from build123d import *

# Parameters (mm, degrees)
CROQUIS1_R              = 17.5
CROQUIS1_R_2            = 12.5
SALIENTE_EXTRUIR1_DEPTH = 40
CROQUIS2_W              = 35
CROQUIS2_H              = 40
SALIENTE_EXTRUIR2_DEPTH = 30
CORTAR_EXTRUIR1_START   = -55
CROQUIS3_R              = 12.5
CORTAR_EXTRUIR1_DEPTH   = 55
CROQUIS4_W              = 26
CROQUIS4_H              = 10
CORTAR_EXTRUIR2_DEPTH   = 55
CROQUIS5_R              = 2.5
CORTAR_EXTRUIR3_DEPTH   = 55
CHAFL_N1_SIZE           = 5
CHAFL_N1_SIZE_2         = 11.23018387
CROQUIS6_W              = 43.374633734
CROQUIS6_H              = 44.438316851
CORTAR_EXTRUIR4_DEPTH   = 5.5
CROQUIS7_R              = 5.5
CORTAR_EXTRUIR5_DEPTH   = 4


with BuildPart() as part:
    # Croquis1 → Saliente-Extruir1 (new body)
    with BuildSketch(Plane(origin=(0, 0, 0), x_dir=(1, 0, 0), z_dir=(0, 1, 0))):
        with Locations(Location((0, 0, 0), (0, 0, 270))):
            Circle(CROQUIS1_R)
        with Locations(Location((0, 0, 0), (0, 0, 270))):
            Circle(CROQUIS1_R_2, mode=Mode.SUBTRACT)
    extrude(amount=SALIENTE_EXTRUIR1_DEPTH)

    # Croquis2 → Saliente-Extruir2 (add)
    with BuildSketch(Plane.XY):
        with Locations((0, 20)):
            Rectangle(CROQUIS2_W, CROQUIS2_H)
    extrude(amount=SALIENTE_EXTRUIR2_DEPTH)

    # Croquis3 → Cortar-Extruir1 (cut)
    with BuildSketch(Plane(origin=(0, 40, 0), x_dir=(1, 0, 0), z_dir=(0, 1, 0)).offset(CORTAR_EXTRUIR1_START)):
        with Locations(Location((0, 0, 0), (0, 0, 270))):
            Circle(CROQUIS3_R)
    extrude(amount=CORTAR_EXTRUIR1_DEPTH, mode=Mode.SUBTRACT)

    # Croquis4 → Cortar-Extruir2 (cut)
    with BuildSketch(Plane(origin=(0, 40, 0), x_dir=(1, 0, 0), z_dir=(0, 1, 0))):
        with Locations((0, -19.512798854)):
            Rectangle(CROQUIS4_W, CROQUIS4_H)
    extrude(amount=-CORTAR_EXTRUIR2_DEPTH, mode=Mode.SUBTRACT)

    # Croquis5 → Cortar-Extruir3 (cut)
    with BuildSketch(Plane.XY.offset(30)):
        with Locations((16, 18)):
            Circle(CROQUIS5_R)
        with Locations((-16, 18)):
            Circle(CROQUIS5_R)
    extrude(amount=-CORTAR_EXTRUIR3_DEPTH, mode=Mode.SUBTRACT)

    # Chaflán1
    # the kernel refuses this chamfer: 11.23018387, 5 mm, written as the material it takes off along each edge
    with BuildSketch(Plane(origin=(17.5, 40, 0), x_dir=(-0.9968798599783936, 0.07893379991777015, 0), z_dir=(0, 0, 1))) as chafl_n1_piece_1:
        Polygon((CHAFL_N1_SIZE * 0.996879859978, CHAFL_N1_SIZE * 0.0789337999178), (-CHAFL_N1_SIZE_2 * 0.0789337999144, CHAFL_N1_SIZE_2 * 0.996879859936), (0, 0), align=None)
    extrude(amount=59.104972531, mode=Mode.SUBTRACT)
    with BuildSketch(Plane(origin=(-17.5, 40, 0), x_dir=(0.9968798599783936, 0.07893379991777015, 0), z_dir=(0, 0, 1))) as chafl_n1_piece_2:
        Polygon((CHAFL_N1_SIZE * 0.996879859978, -CHAFL_N1_SIZE * 0.0789337999178), (-CHAFL_N1_SIZE_2 * 0.0789337999144, -CHAFL_N1_SIZE_2 * 0.996879859936), (0, 0), align=None)
    extrude(amount=59.104972531, mode=Mode.SUBTRACT)
    with BuildSketch(Plane(origin=(0, 40, 0), x_dir=(1, 0, 0), z_dir=(0, 0, 1))) as chafl_n1_piece_3:
        Polygon((17.5 - CHAFL_N1_SIZE, 0), (17.5, -CHAFL_N1_SIZE_2), (17.5, 0), align=None)
    revolve(axis=Axis((0, 40, 0), (0, 1, 0)), revolution_arc=180, mode=Mode.SUBTRACT)

    # Croquis6 → Cortar-Extruir4 (cut)
    with BuildSketch(Plane.XY.offset(30)):
        with Locations((0, 20.325014285)):
            Rectangle(CROQUIS6_W, CROQUIS6_H)
    extrude(amount=-CORTAR_EXTRUIR4_DEPTH, mode=Mode.SUBTRACT)

    # Croquis7 → Cortar-Extruir5 (cut)
    with BuildSketch(Plane.XY.offset(14)):
        with Locations((-16, 18)):
            Circle(CROQUIS7_R)
    cortar_extruir5 = extrude(amount=-CORTAR_EXTRUIR5_DEPTH, mode=Mode.SUBTRACT)

    # Simetría1: Cortar-Extruir5 across plane
    add(cortar_extruir5.mirror(Plane(origin=(0, 0, 0), x_dir=(0, 0, 1), z_dir=(1, 0, 0))), mode=Mode.SUBTRACT)


solid = part.part
For this review, take the finished solid that the model builds, in its own axes (mm). A direction names the side the tool comes from. Round coordinates to 2 decimals unless told otherwise and drop trailing zeros. Order: outer loops, then holes, each group sorted by start corner. A loop starts at its lowest first (then second) coordinate and runs counter-clockwise, first axis right, second up. Notation, with made-up numbers: M 56.25,19.25 L 90.25,19.25 A36 cw 90.25,53.25 Z; hole C 75,66.5 d2. An arc over 180 degrees is marked long. Use a Markdown table: item, result. Add a question column.
Item 1: To check wall thickness, follow line 1 along X through (y, z) = (9.5, 0); line 2 along X through (y, z) = (24.5, 17); line 3 along Y through (x, z) = (-16, 21). State the ranges of each line that lie inside material, in increasing order.
Item 2: Add section A-A, the plane z = 19. Give the boundary of the cut face in (x, y).
Item 3: Mouldability with a two-part tool opening along X and no side actions: class faces 4 (the conical face through (0.31, 36.8, -13.92)), 5 (the flat face through (-13, 20, 20)), 6 (the flat face through (17.5, 8, 12)) as released by +X, released by -X, zero draft, split by the parting line, or undercut.
Item 4: Add section C-C, the plane y = 18. Give the boundary of the cut face in (x, z).
Item 5: Add section D-D, the plane z = 1.5. Give the boundary of the cut face in (x, y), then the cut area to 3 significant figures.
Item 6: Tool access review of faces 1 (the cylindrical face through (-10.5, 17.9, 12)), 2 (the flat face through (-17.5, 8, 12)), 3 (the flat face through (13, 20, 20)): name each direction out of +Z, -Z, +X, -X, +Y, -Y from which nothing blocks a thin tool from reaching the whole face with its end or side.
Item 7: Insertion check: pin 1 (12 mm diameter, centred on x = -9.5, z = 18, fed in from +Y); pin 2 (5.5 mm diameter, centred on x = -13, y = 16.5, fed in from -Z); pin 3 (4.5 mm diameter, centred on x = -16, y = 18, fed in from +Z) (3 decimals); pin 4 (13 mm diameter, centred on x = 6, y = 27.5, fed in from +Z). Each pin has a flat end and moves straight along its axis. Give the tip position at first contact, or say it passes through.
Item 8: Add section B-B, the plane x = 0. Give the boundary of the cut face in (y, z).
Geometry results:
| question | item | result |
|---|---|---|
| 1 | line 1 | x = -17.5 to -12.5, 12.5 to 17.5 |
| 1 | line 2 | x = -17.5 to -13, 13 to 17.5 |
| 1 | line 3 | y = 0 to 15.5, 20.5 to 32.14 |
| 2 | outline | M -17.5,0 L -13,0 L -13,38.88 L -17.5,28.77 L -17.5,20 A2.5 cw long -17.5,16 Z; M 13,0 L 17.5,0 L 17.5,16 A2.5 cw long 17.5,20 L 17.5,28.77 L 13,38.88 Z |
| 3 | face 4 | split by the parting line |
| 3 | face 5 | undercut |
| 3 | face 6 | released by +X |
| 4 | outline | M -13.5,-11.14 A17.5 ccw 13.5,-11.14 L 13.5,10 L 10.5,10 L 10.5,14 L 13.5,14 L 13.5,24.5 L 13,24.5 L 13,14.51 L -13,14.51 L -13,24.5 L -13.5,24.5 L -13.5,14 L -10.5,14 L -10.5,10 L -13.5,10 Z; hole C 0,0 d25 |
| 5 | outline | M -17.5,0 L -12.41,0 L -12.41,40 L -12.5,40 L -17.5,28.77 L -17.5,20 A2.5 cw long -17.5,16 Z; M 12.41,0 L 17.5,0 L 17.5,16 A2.5 cw long 17.5,20 L 17.5,28.77 L 12.5,40 L 12.41,40 Z |
| 5 | area | 317 mm² |
| 6 | face 1 | none |
| 6 | face 2 | +Z, -Z, -X, +Y, -Y |
| 6 | face 3 | +Z, +Y, -Y |
| 7 | pin 1 | stops at y = 40 |
| 7 | pin 2 | stops at z = -14.18 |
| 7 | pin 3 | passes through |
| 7 | pin 4 | stops at z = 14.51 |
| 8 | outline | M 0,-17.5 L 28.77,-17.5 L 40,-12.5 L 0,-12.5 Z; M 0,12.5 L 40,12.5 L 40,14.51 L 0,14.51 Z |
